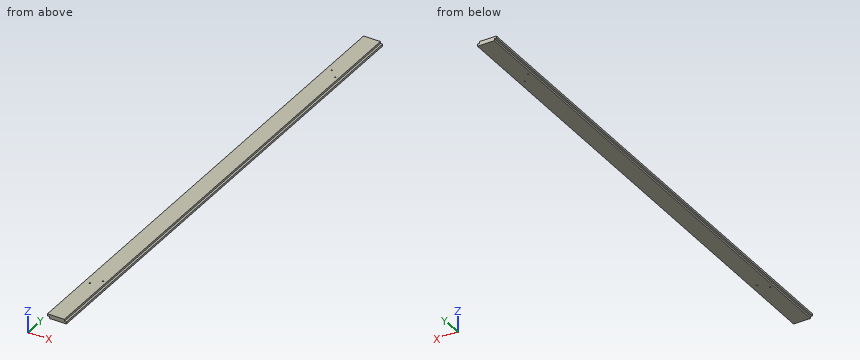
from build123d import *

# Parameters (mm, degrees)
F0_W     = 88.9
F0_H     = 19.05
F1_DEPTH = 1219.2
F2_W     = 47.0931410961
F2_H     = 23.1275351422
F2_W_2   = 44.1598849037
F2_H_2   = 21.9993637201
F3_DEPTH = 2438.401
F4_R     = 3.175
F5_DEPTH = 19.051


with BuildPart() as f1:
    # F0 (on Front) → F1 (new body, symmetric)
    with BuildSketch(Plane.XZ):
        Rectangle(F0_W, F0_H)
    extrude(amount=F1_DEPTH, both=True)

    # F2 (on face) → F3 (cut, through all)
    with BuildSketch(Plane.XZ.offset(1219.2)):
        with Locations((-58.471570548, -11.5637675711)):
            Rectangle(F2_W, F2_H)
        with Locations((57.0049424518, 10.9996818601)):
            Rectangle(F2_W_2, F2_H_2)
    extrude(amount=-F3_DEPTH, mode=Mode.SUBTRACT)

    # F4 (on face) → F5 (cut, through all)
    with BuildSketch(Plane.XY.offset(9.525)):
        with Locations((-19.05, -933.45)):
            Circle(F4_R)
        with Locations((19.05, -895.35)):
            Circle(F4_R)
        with Locations((-19.05, 933.45)):
            Circle(F4_R)
        with Locations((19.05, 895.35)):
            Circle(F4_R)
    extrude(amount=-F5_DEPTH, mode=Mode.SUBTRACT)


solid = f1.part
Build history of the part. All positions in model axes, mm. Give positions to 0.01 mm unless a question says otherwise; leave off trailing zeros. Loops run counter-clockwise (first coordinate to the right, second up) from the corner with the lowest first, then second, coordinate; pieces in that order, holes last. Notation, with made-up numbers: (51.5, 1.25) - (73.5, 1.25) arc R4 ccw to (73.5, 6.25) - close; hole circle Ø9 at (0.5, -21). An arc over 180 degrees is marked (long way). Write item = value, one per line. Start each with the question number.
1) Probe probe 1 along Y at (x, z) = (-19.05, 0) (3 decimals); probe 2 along Y at (x, z) = (19.05, -4.5) (3 decimals); probe 3 along X at (y, z) = (-933.45, -3) (3 decimals). List the from-to ranges inside material, lowest first. Write a range as from..to.
2) Band-saw the part on B-B on y = 234.5. Give the cut face in (x, z) (3 decimals), plus the area to 3 significant figures.
3) Band-saw the part on A-A on z = 6.5. Give the cut face in (x, y) (3 decimals), plus the area to 3 significant figures.
4) Drop flat-ended pins along their axis: pin 1 Ø3 at (y, z) = (45, -2.5) entering from -X (3 decimals); pin 2 Ø10.5 at (y, z) = (-46, 4) entering from +X; pin 3 Ø3 at (x, y) = (41, -174.5) entering from +Z; pin 4 Ø10.5 at (x, y) = (-41, -506.5) entering from -Z. Give the stop position or say it passes through.
Final values:
q1.probe_1 = -1219.2..-936.625, -930.275..930.275, 936.625..1219.2
q1.probe_2 = -1219.2..-898.525, -892.175..892.175, 898.525..1219.2
q1.probe_3 = -34.925..-22.225, -15.875..44.45
q2.outline = (-44.45, 0) - (-34.925, 0) - (-34.925, -9.525) - (44.45, -9.525) - (44.45, 0) - (34.925, 0) - (34.925, 9.525) - (-44.45, 9.525) - close
q2.area = 1,510 mm²
q3.outline = (-44.45, -1219.2) - (34.925, -1219.2) - (34.925, 1219.2) - (-44.45, 1219.2) - close; hole circle Ø6.35 at (-19.05, -933.45); hole circle Ø6.35 at (-19.05, 933.45); hole circle Ø6.35 at (19.05, -895.35); hole circle Ø6.35 at (19.05, 895.35)
q3.area = 193,000 mm²
q4.pin_1 = -34.925
q4.pin_2 = 44.45
q4.pin_3 = 0
q4.pin_4 = 0
